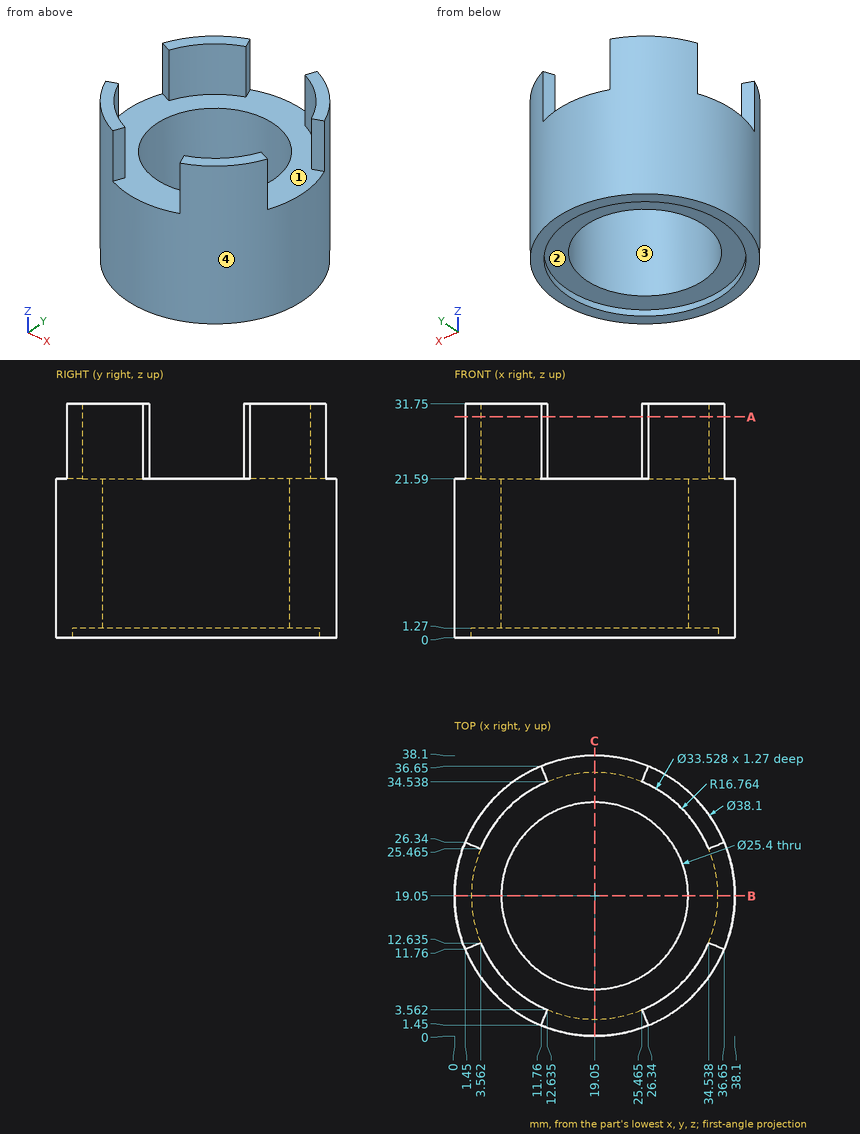
The figure shows three views and two pictorial views of one solid part (mm, origin at its lowest corner). Answer the questions. A direction names the side the tool comes from. Give positions to 0.01 mm unless a question says otherwise; leave off trailing zeros. Write each loop counter-clockwise with the first axis right and the second up, starting at its lowest first coordinate (ties: lowest second). Pieces come first, ordered by that corner, then holes. Notation, with made-up numbers: (58, 2) -> (96, 2) arc R7 ccw to (96, 12) -> close; hole circle Ø8 at (-24, 39). An arc over 180 degrees is marked (long way). Write each question's results on one line, items separated by ' | '.
1. Straight lines are drawn through the part: L1, parallel to Y at x = 19, z = 9; L2, parallel to Z at x = 23.5, y = 6; L3, parallel to Y at x = 29, z = 3.5 (1 decimal). For each, find the intervals that lie inside material, in ascending order.
Data:
L1: 0 to 6.35, 31.75 to 38.1 | L2: 1.27 to 21.59 | L3: 2.8 to 11.2, 26.9 to 35.3
2. Find section B-B on y = 19.05. Determine the outline of the cut face in (x, z), and give its area (3 significant figures).
Data:
outline: (0, 0) -> (2.29, 0) -> (2.29, 1.27) -> (6.35, 1.27) -> (6.35, 21.59) -> (0, 21.59) -> close; (31.75, 1.27) -> (35.81, 1.27) -> (35.81, 0) -> (38.1, 0) -> (38.1, 21.59) -> (31.75, 21.59) -> close | area: 264 mm^2
3. A tool of negligible diameter and unlimited length cuts with its end or side. For the marked faces 1 and 2, from which of +Z, -Z, +X, -X, +Y, -Y can it reach the whole face along a straight path? Write none if from no direction.
Data:
face 1: +Z | face 2: -Z
4. Find section A-A on z = 30. Give the number of separate pieces and of enclosed holes in the cut face, and give its area (3 significant figures).
Data:
separate pieces: 4 | enclosed holes: 0 | area: 129 mm^2
5. Determine the mould class of the marked faces 3 and 4 for opening direction X: +X half, -X half, draft (parallel to the pull), parting line (faces both ways), or undercut.
Data:
face 3: undercut | face 4: parting line
6. Each of these flat-tipped pins is pushed along its axis until it touches: pin 1 Ø5 at (y, z) = (23, 7.5) entering from -X (1 decimal); pin 2 Ø4 at (x, z) = (33, 5.5) entering from +Y (1 decimal); pin 3 Ø10 at (y, z) = (25, 17.5) entering from +X; pin 4 Ø8 at (x, y) = (32.5, 27.5) entering from -Z. Where does it stop, or does it pass through?
Data:
pin 1: x = 0.1 | pin 2: y = 33.9 | pin 3: x = 38.08 | pin 4: z = 0
